from build123d import *

# Parameters (mm, degrees)
F0_R     = 2.6
F1_DEPTH = 11.5
F3_W     = 8.5
F3_H     = 10
F3_H_2   = 9.3
F4_DEPTH = 2.15


with BuildPart() as f1:
    # F0 (on Top) → F1 (new body)
    with BuildSketch(Plane.XY):
        with BuildLine():
            ThreePointArc((-4.23999152, -6.783986432), (3.8781482591, -6.99713985), (8, 0))
            ThreePointArc((8, 0), (6.99713985, 3.8781482591), (4.23999152, 6.783986432))
            ThreePointArc((4.23999152, 6.783986432), (-6.783986432, 4.23999152), (-4.23999152, -6.783986432))
        make_face()
        Circle(F0_R, mode=Mode.SUBTRACT)
        with BuildLine():
            ThreePointArc((4.23999152, 6.783986432), (6.99713985, 3.8781482591), (8, 0))
            ThreePointArc((8, 0), (3.8781482591, -6.99713985), (-4.23999152, -6.783986432))
            Line((-4.23999152, -6.783986432), (11.76000848, -16.783986432))
            ThreePointArc((11.76000848, -16.783986432), (9.216013568, -5.76000848), (20.23999152, -3.216013568))
            Line((20.23999152, -3.216013568), (4.23999152, 6.783986432))
        make_face()
        with BuildLine():
            ThreePointArc((24, -10), (22.99713985, -6.1218517409), (20.23999152, -3.216013568))
            ThreePointArc((20.23999152, -3.216013568), (9.216013568, -5.76000848), (11.76000848, -16.783986432))
            ThreePointArc((11.76000848, -16.783986432), (19.8781482591, -16.99713985), (24, -10))
        make_face()
        with Locations((16, -10)):
            Circle(F0_R, mode=Mode.SUBTRACT)
    extrude(amount=F1_DEPTH)

    # F3 (on mid) → F4 (cut, symmetric)
    with BuildSketch(Plane.XY.offset(5.75)):
        with Locations((0, -9.65)):
            Rectangle(F3_W, F3_H)
        Rectangle(F3_W, F3_H_2)
        with Locations((16, -19.65)):
            Rectangle(F3_W, F3_H)
        with Locations((16, -10)):
            Rectangle(F3_W, F3_H_2)
    extrude(amount=F4_DEPTH, both=True, mode=Mode.SUBTRACT)


solid = f1.part
Could you check a few things on this model? Use its own coordinates, in mm. A direction names the side the tool comes from. Round coordinates to 2 decimals unless told otherwise and drop trailing zeros. Loops run counter-clockwise (first coordinate to the right, second up) from the corner with the lowest first, then second, coordinate; pieces in that order, holes last. Notation, with made-up numbers: (78, 75.25) -> (82, 75.25) arc R13 cw to (82, 86.25) -> close; hole circle Ø4 at (-16, 33). An arc over 180 degrees is marked (long way). Use CSV: the item, a comma, the result in double quotes.
(1) If I drill on probe 1 along Z at (x, y) = (2.5, -6.5); probe 2 along Y at (x, z) = (0, 9.4); probe 3 along X at (y, z) = (0, 3.25), over which ranges is the centre line in solid material (lowest first)? Write a range as [from, to].
Return value:
probe 1,"z = [0, 3.6], [7.9, 11.5]"
probe 2,"y = [-9.43, -2.6], [2.6, 8]"
probe 3,"x = [-8, -2.6], [2.6, 15.09]"
(2) Suppose I cut it at B-B on x = 0.5. Write out the boundary of the cut face in (y, z).
Return value:
outline,"(-9.75, 0) -> (-2.55, 0) -> (-2.55, 3.6) -> (-9.75, 3.6) -> close; (-9.75, 7.9) -> (-2.55, 7.9) -> (-2.55, 11.5) -> (-9.75, 11.5) -> close; (2.55, 0) -> (7.98, 0) -> (7.98, 11.5) -> (2.55, 11.5) -> (2.55, 7.9) -> (4.65, 7.9) -> (4.65, 3.6) -> (2.55, 3.6) -> close"
(3) Suppose I cut it at C-C on y = 0. Write out the boundary of the cut face in (x, z), plus the area to 3 significant figures.
Return value:
outline,"(-8, 0) -> (-2.6, 0) -> (-2.6, 3.6) -> (-4.25, 3.6) -> (-4.25, 7.9) -> (-2.6, 7.9) -> (-2.6, 11.5) -> (-8, 11.5) -> close; (2.6, 0) -> (15.09, 0) -> (15.09, 11.5) -> (2.6, 11.5) -> (2.6, 7.9) -> (4.25, 7.9) -> (4.25, 3.6) -> (2.6, 3.6) -> close"
area,"192 mm²"
(4) For faces 1 (the flat face through (8, -5, 0)), 2 (the flat face through (11.75, -11, 6)), which set-ups out of +Z, -Z, +X, -X, +Y, -Y let a thin tool reach every point of the face, with its end or its side?
Return value:
face 1,"-Z, +X, -X, +Y, -Y"
face 2,"-Y"
(5) Suppose I cut it at D-D on z = 4. Write out the boundary of the cut face in (x, y).
Return value:
outline,"(-4.25, -6.78) -> (-4.25, 4.65) -> (4.25, 4.65) -> (4.25, -12.09) -> (11.75, -16.78) -> (11.75, -5.35) -> (20.25, -5.35) -> (20.25, -16.78) arc R8 ccw to (20.24, -3.22) -> (4.24, 6.78) arc R8 ccw to start"
(6) If we mould it in two halves opening along Y, with no side actions, what happens to faces 3 (the flat face through (4.25, -4, 6)), 4 (the flat face through (16, -5.35, 6)), 5 (the cylindrical face through (18.4, -11, 9.7))? For each: +Y half, -Y half, draft (parallel to the pull), parting line (faces both ways), or undercut.
Return value:
face 3,"draft"
face 4,"-Y half"
face 5,"undercut"
(7) Will these pins go through, and if not, where does the flat tip stop? pin 1 Ø2 at (x, z) = (-0.5, 6) entering from -Y; pin 2 Ø1 at (y, z) = (-10, 6.5) entering from -X; pin 3 Ø6 at (x, z) = (-4, 4) entering from +Y; pin 4 Ø4.5 at (x, y) = (15.5, -11) entering from -Z.
Return value:
pin 1,"stops at y = 4.65"
pin 2,"stops at x = 4.25"
pin 3,"stops at y = 7.94"
pin 4,"stops at z = 0"
